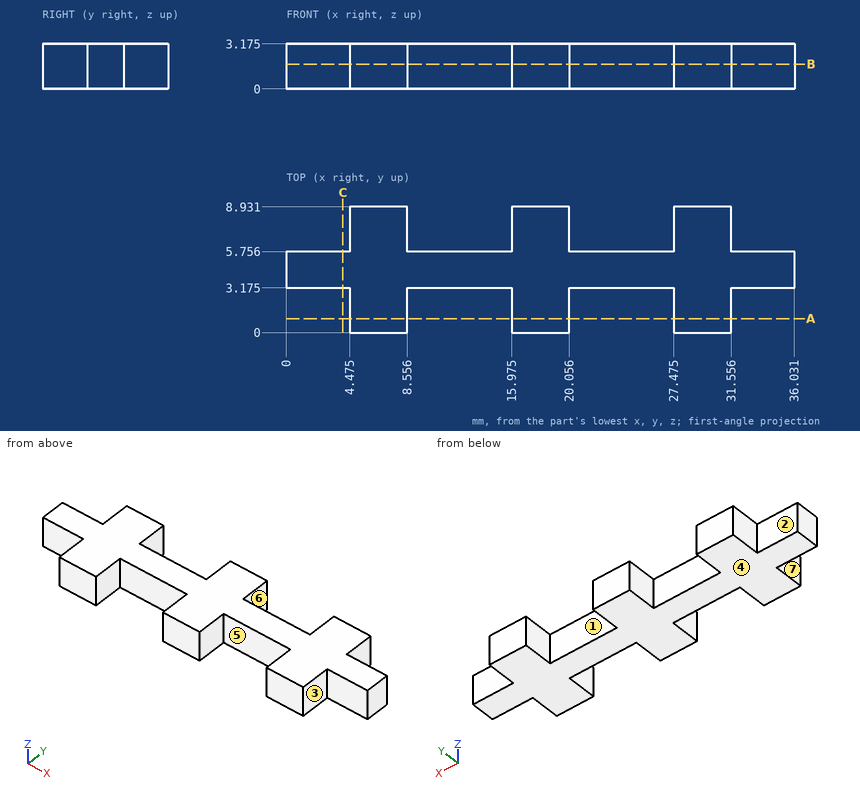
Input: dimensioned drawing with shaded views. Units: mm. Origin: part minimum x, y, z. A direction names the side the tool comes from. Give positions to 0.01 mm unless a question says otherwise; leave off trailing zeros. Order: outer loops, then holes, each group sorted by start corner. A loop starts at its lowest first (then second) coordinate and runs counter-clockwise, first axis right, second up.
(1) Section query C-C (x = 4). Return the cut outline in (y, z) (1 decimal).
(2) Section query B-B (z = 1.75). Return the cut outline in (x, y) (1 decimal), plus the area to 3 significant figures.
(3) Access query for the marked faces 4, 5, 6 and 7. Directions: +Z, -Z, +X, -X, +Y, -Y. A direction counts if a zero-diameter tool reaches every point of the face in a straight line with its end or side. Return the directions, or none.
(4) Material intervals for line 1 along X through (y, z) = (7.5, 2.9) (1 decimal); line 2 along Y through (x, z) = (2.5, 1.15) (1 decimal), sorted ascending.
(5) Contact query for flat-ended pins moving along their axis: P1, Ø1.6, axis at x = 12.5, z = 1, coming from the +Y side; P2, Ø1, axis at x = 32, z = 0.5, coming from the +Y side; P3, Ø1.6, axis at y = 8, z = 1.5, coming from the -X side (3 decimals); P4, Ø1.6, axis at y = 7.5, z = 1.5, coming from the +X side. Output: stop coordinate, or through.
(6) Section query A-A (y = 1). Return the cut outline in (x, z) (1 decimal).
(7) Pull-direction query (X, two-part tool) for the marked faces 1, 2 and 3; classes: +X half, -X half, draft (parallel to the pull), parting line (faces both ways), or undercut.
Outcome:
1. outline: (3.2, 0) - (5.8, 0) - (5.8, 3.2) - (3.2, 3.2) - close
2. outline: (0, 3.2) - (4.5, 3.2) - (4.5, 0) - (8.6, 0) - (8.6, 3.2) - (16, 3.2) - (16, 0) - (20.1, 0) - (20.1, 3.2) - (27.5, 3.2) - (27.5, 0) - (31.6, 0) - (31.6, 3.2) - (36, 3.2) - (36, 5.8) - (31.6, 5.8) - (31.6, 8.9) - (27.5, 8.9) - (27.5, 5.8) - (20.1, 5.8) - (20.1, 8.9) - (16, 8.9) - (16, 5.8) - (8.6, 5.8) - (8.6, 8.9) - (4.5, 8.9) - (4.5, 5.8) - (0, 5.8) - close
2. area: 171 mm2
3. face 4: -Z, +X, -X, +Y, -Y
3. face 5: +Z, -Z, -Y
3. face 6: +Z, -Z, +Y
3. face 7: +Z, -Z, -X, -Y
4. line 1: x = 4.5 to 8.6, 16 to 20.1, 27.5 to 31.6
4. line 2: y = 3.2 to 5.8
5. P1: stops at y = 5.76
5. P2: stops at y = 8.93
5. P3: stops at x = 4.475
5. P4: stops at x = 31.56
6. outline: (4.5, 0) - (8.6, 0) - (8.6, 3.2) - (4.5, 3.2) - close; (16, 0) - (20.1, 0) - (20.1, 3.2) - (16, 3.2) - close; (27.5, 0) - (31.6, 0) - (31.6, 3.2) - (27.5, 3.2) - close
7. face 1: undercut
7. face 2: draft
7. face 3: +X half
